Could you check a few things on this model? Use its own coordinates, in mm. A direction names the side the tool comes from. Give positions to 0.01 mm unless a question says otherwise; leave off trailing zeros. Write each loop counter-clockwise with the first axis right and the second up, starting at its lowest first coordinate (ties: lowest second). Pieces come first, ordered by that corner, then holes. Notation, with made-up numbers: (64, 45.25) -> (69, 45.25) arc R17 cw to (69, 63.25) -> close; hole circle Ø3 at (10, -23.75). An arc over 180 degrees is marked (long way). One line per question, with ' | ' between items.
from build123d import *

# Parameters (mm, degrees)
CYLINDER002_R     = 1.75
CYLINDER002_DEPTH = 10
CYLINDER003_R     = 3
CYLINDER003_DEPTH = 3


with BuildPart() as cone:
    # Cone → Cone (revolve)
    with BuildSketch(Plane(origin=(0, 0, 9), x_dir=(1, 0, 0), z_dir=(0, -1, 0))):
        Polygon((0, 0), (1, 0), (3, 2), (0, 2), align=None)
    revolve(axis=Axis((0, 0, 9), (0, 0, 1)))


with BuildPart() as cylinder002:
    # Cylinder002 → Cylinder002 (new body)
    with BuildSketch(Plane.XY):
        Circle(CYLINDER002_R)
    extrude(amount=CYLINDER002_DEPTH)


with BuildPart() as fusion002:
    # Cylinder003 → Cylinder003 (new body)
    with BuildSketch(Plane.XY.offset(11)):
        Circle(CYLINDER003_R)
    extrude(amount=CYLINDER003_DEPTH)

    # Fusion002: union Cone, Cylinder002
    add(cone.part)
    add(cylinder002.part)


solid = fusion002.part
Q1. Imagine slicing it at C-C on z = 11.25. Please give me the cut outline in (x, y).
Answer below:
outline: circle Ø6 at (0, 0)
Q2. If I drill on line 1 along X through (y, z) = (0.05, 8.5); line 2 along Z through (x, y) = (-2.3, -1.8), over which ranges is the centre line in solid material (lowest first)?
Answer below:
line 1: x = -1.75 to 1.75 | line 2: z = 10.92 to 14
Q3. Imagine slicing it at D-D on z = 4.75. Please give me the cut outline in (x, y).
Answer below:
outline: circle Ø3.5 at (0, 0)
Q4. On a 3-axis mill with a long thin cutter (end or side, diameter ignored), from which of +Z, -Z, +X, -X, +Y, -Y can I reach the whole of each face in a straight line? I mean faces 1 (the flat face through (0, 0, 14)), 2 (the cylindrical face through (1.617, -0.67, 4.807)). Say none if no direction works.
Answer below:
face 1: +Z, +X, -X, +Y, -Y | face 2: -Z
Q5. Imagine slicing it at A-A on x = 0. Please give me the cut outline in (y, z).
Answer below:
outline: (-3, 11) -> (-1.75, 9.75) -> (-1.75, 0) -> (1.75, 0) -> (1.75, 9.75) -> (3, 11) -> (3, 14) -> (-3, 14) -> close
Q6. Will these pins go through, and if not, where does the flat tip stop? pin 1 (2 mm diameter, centred on y = -2, z = 4.5, fed in from +X); pin 2 (3 mm diameter, centred on y = -0.5, z = 9, fed in from +X).
Answer below:
pin 1: stops at x = 1.44 | pin 2: stops at x = 2.47
